Build history of the part. All positions in model axes, mm. Face numbers are marked on the shaded views. A direction names the side the tool comes from. Coordinates: 2 decimals unless noted, no trailing zeros. Order: outer loops, then holes, each group sorted by start corner. A loop starts at its lowest first (then second) coordinate and runs counter-clockwise, first axis right, second up. Notation, with made-up numbers: (-7, -11.75) - (51, -11.75) arc R28 ccw to (51, 8.25) - close; hole circle Ø8 at (72.25, -12). An arc over 180 degrees is marked (long way). Write each question's results on one line, items separated by ' | '.
from build123d import *

# Parameters (mm, degrees)
SKETCH2_W                = 4
SKETCH2_H                = 15
BOSS_EXTRUDE1_DEPTH      = 10
BOSS_EXTRUDE1_2_DEPTH    = 10
BOSS_EXTRUDE2_DEPTH      = 7.5
BOSS_EXTRUDE2_DEPTH_BACK = 7.5
SKETCH3_W                = 30
SKETCH3_H                = 5


with BuildPart() as part:
    # Sketch2 → Boss-Extrude1 (new body)
    with BuildSketch(Plane(origin=(0, 0, 0), x_dir=(1, 0, 0), z_dir=(0, 1, 0))):
        with Locations((-13, 0)):
            Rectangle(SKETCH2_W, SKETCH2_H)
    extrude(amount=-BOSS_EXTRUDE1_DEPTH)



with BuildPart() as body_2:
    # Sketch2 → Boss-Extrude1 2 (new body)
    with BuildSketch(Plane(origin=(0, 0, 0), x_dir=(1, 0, 0), z_dir=(0, 1, 0))):
        with Locations((13, 0)):
            Rectangle(SKETCH2_W, SKETCH2_H)
    extrude(amount=-BOSS_EXTRUDE1_2_DEPTH)


with BuildPart() as part_1:
    add(part.part)

    add(body_2.part)  # Boss-Extrude2 merges body 2
    # Sketch3 → Boss-Extrude2 (add, two sides: drawn at the far end of the back side and taken through both)
    with BuildSketch(Plane.XY.offset(-BOSS_EXTRUDE2_DEPTH_BACK)):
        with Locations((0, 2.5)):
            Rectangle(SKETCH3_W, SKETCH3_H)
    extrude(amount=BOSS_EXTRUDE2_DEPTH + BOSS_EXTRUDE2_DEPTH_BACK)


solid = part_1.part
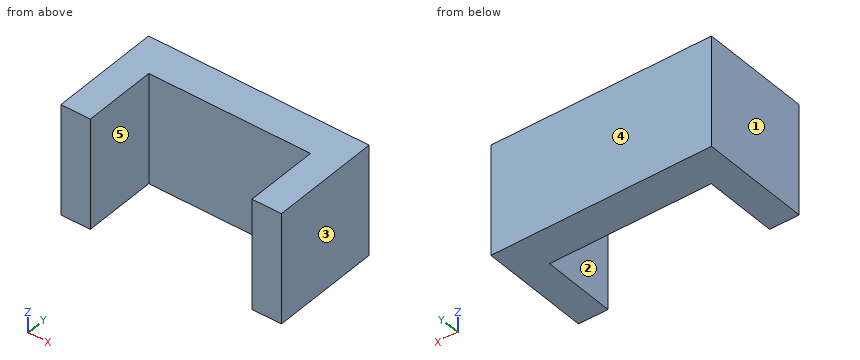
1. Tool access for the marked faces 1 and 2: list every direction of +Z, -Z, +X, -X, +Y, -Y with a clear straight run to the whole face (end or side of a thin tool).
Solved:
face 1: +Z, -Z, -X, +Y, -Y | face 2: +Z, -Z, -Y
2. Two-plate mould, pull along X, no slides. Class the marked faces 3, 4 and 5: +X half, -X half, draft (parallel to the pull), parting line (faces both ways), or undercut.
Solved:
face 3: +X half | face 4: draft | face 5: undercut
3. Drop a flat-ended pin along its axis: pin 1 Ø6 at (x, z) = (-7.5, -0.5) entering from -Y. Give the stop position or say it passes through.
Solved:
pin 1: stops at y = 0
4. Band-saw the part on B-B on z = 3.25. Give the cut face in (x, y).
Solved:
outline: (-15, -10) - (-11, -10) - (-11, 0) - (11, 0) - (11, -10) - (15, -10) - (15, 5) - (-15, 5) - close
5. Band-saw the part on A-A on y = -1.5. Give the cut face in (x, z), then the cut area to 3 significant figures.
Solved:
outline: (-15, -7.5) - (-11, -7.5) - (-11, 7.5) - (-15, 7.5) - close; (11, -7.5) - (15, -7.5) - (15, 7.5) - (11, 7.5) - close | area: 120 mm2
6. Band-saw the part on C-C on x = 4.25. Give the cut face in (y, z).
Solved:
outline: (0, -7.5) - (5, -7.5) - (5, 7.5) - (0, 7.5) - close
7. Probe line 1 (X direction, y = -2.75, z = -6.5); line 2 (Y direction, x = 3, z = -0.75). List the from-to ranges inside material, lowest first.
Solved:
line 1: x = -15 to -11, 11 to 15 | line 2: y = 0 to 5
